Work out the finished part from the listing and answer in its coordinate system (mm). Round coordinates to 2 decimals unless told otherwise and drop trailing zeros. Order: outer loops, then holes, each group sorted by start corner. A loop starts at its lowest first (then second) coordinate and runs counter-clockwise, first axis right, second up. Notation, with made-up numbers: (17.25, 33) - (49.25, 33) arc R29 ccw to (49.25, 59) - close; hole circle Ø5 at (76, -5.5). An arc over 180 degrees is marked (long way). Use CSV: the item, a comma, the result in double quotes.
Autodesk Inventor part; units mm, degrees
ref_plane "YZ Plane" through (0, 0, 0) normal (1, 0, 0) x (0, 1, 0)
ref_plane "XZ Plane" through (0, 0, 0) normal (0, 1, 0) x (-1, 0, 0)
ref_plane "XY Plane" through (0, 0, 0) normal (0, 0, 1) x (1, 0, 0)
sketch "Sketch1" plane through (0, 0, 0) normal (0, 1, 0) x (-1, 0, 0)
  line L0 (-50, 37.5) -> (50, 37.5)
  line L1 (50, 37.5) -> (50, -37.5)
  line L2 (50, -37.5) -> (-50, -37.5)
  line L3 (-50, -37.5) -> (-50, 37.5)
  line L4 (-50, 37.5) -> (50, -37.5) construction
  line L5 (50, 37.5) -> (-50, -37.5) construction
  line L6 (50, 0) -> (10, 0)
  circle A0 centre (10, 0) radius 27.5
  point P0 (0, 0)
  dimension "d0" = 100
  dimension "d1" = 75
  dimension "d2" = 40
  dimension "d3" = 55
extrude "Extrusion1" add sketch "Sketch1" along normal blind 10
sketch "Sketch2" plane through (0, 10, 0) normal (0, 1, 0) x (1, 0, 0)
  line L0 (50, 37.5) -> (-50, 37.5)
  line L1 (-50, -37.5) -> (50, -37.5)
  line L2 (50, 37.5) -> (40, 37.5)
  line L3 (40, 37.5) -> (40, -37.5)
  line L4 (40, -37.5) -> (50, -37.5)
  line L5 (50, -37.5) -> (50, 37.5)
  line L6 (45, 37.5) -> (45, 0)
  line L7 (45, 0) -> (45, -37.5)
  circle A0 centre (45, 18.75) radius 3.3
  circle A1 centre (45, -18.75) radius 3.3
  point P0 (0, 0)
  dimension "d6" = 10
  dimension "d7" = 6.6
  dimension "d8" = 6.6
extrude "Extrusion2" cut sketch "Sketch2" against normal up to surface (10 mm away) contours A0 L6 | L6 A0 | A1 L7 | L7 A1
fillet "Fillet1" radius 1 2 edges at (0, 10, 37.5) (0, 10, -37.5)
properties part number "blok_łożyska"
(1) Find section D-D (y = 7). Determine the outline of the cut face in (x, z).
Findings below:
outline,"(-50, -37.5) - (50, -37.5) - (50, 37.5) - (-50, 37.5) - close; hole circle Ø55 at (-10, 0); hole circle Ø6.6 at (45, -18.75); hole circle Ø6.6 at (45, 18.75)"
(2) Find section A-A (x = 45). Determine the outline of the cut face in (y, z), and give its area (3 significant figures).
Findings below:
outline,"(0, -37.5) - (9, -37.5) arc R1 ccw to (10, -36.5) - (10, -22.05) - (0, -22.05) - close; (0, -15.45) - (10, -15.45) - (10, 15.45) - (0, 15.45) - close; (0, 22.05) - (10, 22.05) - (10, 36.5) arc R1 ccw to (9, 37.5) - (0, 37.5) - close"
area,"618 mm²"
(3) Find the intervals of material crossed by L1, parallel to Z at x = 45, y = 6.25; L2, parallel to X at y = 6.75, z = -18.75; L3, parallel to X at y = 7.75, z = 18, in increasing order. Write a range as from..to.
Findings below:
L1,"z = -37.5..-22.05, -15.45..15.45, 22.05..37.5"
L2,"x = -50..-30.12, 10.12..41.7, 48.3..50"
L3,"x = -50..-30.79, 10.79..41.79, 48.21..50"
(4) Find section C-C (x = -10). Determine the outline of the cut face in (y, z), and give its area (3 significant figures).
Findings below:
outline,"(0, -37.5) - (9, -37.5) arc R1 ccw to (10, -36.5) - (10, -27.5) - (0, -27.5) - close; (0, 27.5) - (10, 27.5) - (10, 36.5) arc R1 ccw to (9, 37.5) - (0, 37.5) - close"
area,"200 mm²"
(5) This flat-tipped pin is pushed along its axis until it touches: pin 1 (4 mm diameter, centred on x = 45, z = -18.75, fed in from +Y). Where does it stop, or does it pass through?
Findings below:
pin 1,"passes through"
(6) Find section B-B (z = 0). Determine the outline of the cut face in (x, y).
Findings below:
outline,"(-50, 0) - (-37.5, 0) - (-37.5, 10) - (-50, 10) - close; (17.5, 0) - (50, 0) - (50, 10) - (17.5, 10) - close"
(7) The mould has two halves that part along X. Classify faces 1 (the cylindrical face through (11.823, 4.93, 16.733)), 2 (the flat face through (-50, 5, 1)), 3 (the flat face through (12, 0, 17)), 4 (the cylindrical face through (41.703, 5.07, 18.605)): released by +X, released by -X, zero draft, split by the parting line, or undercut.
Findings below:
face 1,"undercut"
face 2,"released by -X"
face 3,"zero draft"
face 4,"undercut"
